Geometry check sheet. Reference: the model listing, model coordinates, mm. A direction names the side the tool comes from. Give positions to 0.01 mm unless a question says otherwise; leave off trailing zeros. Order: outer loops, then holes, each group sorted by start corner. A loop starts at its lowest first (then second) coordinate and runs counter-clockwise, first axis right, second up. Notation, with made-up numbers: M 53,-26 L 87,-26 A12 cw 87,-15 Z; hole C 56.5,71.5 d10. An arc over 180 degrees is marked long. One line per question, with ' | ' between items. Start each with the question number.
from build123d import *
from build123d.topology import SkipClean

# Parameters (mm, degrees)
EXTRUDE_1_DEPTH     = 3
SKETCH_4_W          = 70
SKETCH_4_H          = 3
EXTRUDE_2_DEPTH     = 9
CUT_EXTRUDE_1_REACH = 88.319
FILLET_1_R          = 1
EXTRUDE_3_DEPTH     = 2


with BuildPart() as part:
    # ｽｹｯﾁ2 → ﾎﾞｽ - 押し出し1 (new body)
    with BuildSketch(Plane(origin=(0, 0, 0), x_dir=(1, 0, 0), z_dir=(0, 1, 0))):
        with BuildLine():
            Line((70, 7.6), (40, 7.6))
            Line((40, 7.6), (40, 4.4))
            Line((40, 4.4), (70, 4.4))
            Line((70, 4.4), (84.5, 4.4))
            ThreePointArc((84.5, 4.4), (84.853553391, 4.253553391), (85, 3.9))
            Line((85, 3.9), (85, 0.5))
            ThreePointArc((85, 0.5), (84.853553391, 0.146446609), (84.5, 0))
            Line((84.5, 0), (83.316300355, 0))
            ThreePointArc((83.316300355, 0), (77.25, 2), (71.183699645, 0))
            Line((71.183699645, 0), (70, 0))
            Line((70, 0), (62, 0))
            Line((62, 0), (62, -0.949194177))
            ThreePointArc((62, -0.949194177), (61.80461807, -1.345688605), (61.371168675, -1.432311647))
            Line((61.371168675, -1.432311647), (56, 0))
            Line((56, 0), (0.5, 0))
            ThreePointArc((0.5, 0), (0.146446609, 0.146446609), (0, 0.5))
            Line((0, 0.5), (0, 11.5))
            ThreePointArc((0, 11.5), (0.146446609, 11.853553391), (0.5, 12))
            Line((0.5, 12), (70, 12))
            Line((70, 12), (71.183699645, 12))
            ThreePointArc((71.183699645, 12), (77.25, 10), (83.316300355, 12))
            Line((83.316300355, 12), (84.5, 12))
            ThreePointArc((84.5, 12), (84.853553391, 11.853553391), (85, 11.5))
            Line((85, 11.5), (85, 8.1))
            ThreePointArc((85, 8.1), (84.853553391, 7.746446609), (84.5, 7.6))
            Line((84.5, 7.6), (70, 7.6))
        make_face()
    extrude(amount=EXTRUDE_1_DEPTH)

    # ｽｹｯﾁ4 → ﾎﾞｽ - 押し出し2 (add)
    with BuildSketch(Plane(origin=(0, 3, 0), x_dir=(1, 0, 0), z_dir=(0, 1, 0))):
        with Locations((35, 9.1)):
            Rectangle(SKETCH_4_W, SKETCH_4_H)
    extrude(amount=EXTRUDE_2_DEPTH)

    # ｽｹｯﾁ5 → ｶｯﾄ - 押し出し1 (cut, up to next)
    with BuildSketch(Plane.XY.offset(-7.6), mode=Mode.PRIVATE) as cut_extrude_1_sk1:
        with BuildLine():
            ThreePointArc((64.370652174, 9.924925734), (63.8, 8.7), (64.370652174, 7.475074266))
            ThreePointArc((64.370652174, 7.475074266), (64.782233047, 6.932233047), (65.325074266, 6.520652174))
            ThreePointArc((65.325074266, 6.520652174), (66.55, 5.95), (67.774925734, 6.520652174))
            ThreePointArc((67.774925734, 6.520652174), (68.317766953, 6.932233047), (68.729347826, 7.475074266))
            ThreePointArc((68.729347826, 7.475074266), (69.3, 8.7), (68.729347826, 9.924925734))
            ThreePointArc((68.729347826, 9.924925734), (68.317766953, 10.467766953), (67.774925734, 10.879347826))
            ThreePointArc((67.774925734, 10.879347826), (66.55, 11.45), (65.325074266, 10.879347826))
            ThreePointArc((65.325074266, 10.879347826), (64.782233047, 10.467766953), (64.370652174, 9.924925734))
        make_face()
    cut_extrude_1_tool1 = extrude(cut_extrude_1_sk1.sketch, amount=-CUT_EXTRUDE_1_REACH, mode=Mode.PRIVATE) & part.part
    # ｽｹｯﾁ5 → ｶｯﾄ - 押し出し1 (cut, up to next)
    with BuildSketch(Plane.XY.offset(-7.6), mode=Mode.PRIVATE) as cut_extrude_1_sk2:
        with BuildLine():
            ThreePointArc((5.629347826, 7.475074266), (6.2, 8.7), (5.629347826, 9.924925734))
            ThreePointArc((5.629347826, 9.924925734), (5.217766953, 10.467766953), (4.674925734, 10.879347826))
            ThreePointArc((4.674925734, 10.879347826), (3.45, 11.45), (2.225074266, 10.879347826))
            ThreePointArc((2.225074266, 10.879347826), (1.682233047, 10.467766953), (1.270652174, 9.924925734))
            ThreePointArc((1.270652174, 9.924925734), (0.7, 8.7), (1.270652174, 7.475074266))
            ThreePointArc((1.270652174, 7.475074266), (1.682233047, 6.932233047), (2.225074266, 6.520652174))
            ThreePointArc((2.225074266, 6.520652174), (3.45, 5.95), (4.674925734, 6.520652174))
            ThreePointArc((4.674925734, 6.520652174), (5.217766953, 6.932233047), (5.629347826, 7.475074266))
        make_face()
    cut_extrude_1_tool2 = extrude(cut_extrude_1_sk2.sketch, amount=-CUT_EXTRUDE_1_REACH, mode=Mode.PRIVATE) & part.part
    add(cut_extrude_1_tool1.solids().sort_by_distance((66.55, 8.7, -7.6))[0], mode=Mode.SUBTRACT)
    add(cut_extrude_1_tool2.solids().sort_by_distance((3.45, 8.7, -7.6))[0], mode=Mode.SUBTRACT)

    # ﾌｨﾚｯﾄ1
    fillet_1_edges = [part.edges().sort_by_distance(p)[0] for p in [
        (70, 12, -9.1),
        (0, 12, -9.1),
    ]]
    fillet(fillet_1_edges, radius=FILLET_1_R)

    # ｽｹｯﾁ6 → ﾎﾞｽ - 押し出し3 (add)
    with SkipClean():  # the faces are left unmerged after this step: merging them gives an invalid solid
        with BuildSketch(Plane.XY.offset(-7.6)):
            with BuildLine():
                Line((1.85, 9.85), (1.85, 7.55))
                ThreePointArc((1.85, 7.55), (1.946690123, 7.002223209), (2.225074266, 6.520652174))
                ThreePointArc((2.225074266, 6.520652174), (1.682233047, 6.932233047), (1.270652174, 7.475074266))
                ThreePointArc((1.270652174, 7.475074266), (0.7, 8.7), (1.270652174, 9.924925734))
                ThreePointArc((1.270652174, 9.924925734), (1.682233047, 10.467766953), (2.225074266, 10.879347826))
                ThreePointArc((2.225074266, 10.879347826), (1.946690123, 10.397776791), (1.85, 9.85))
            make_face()
            with BuildLine():
                Line((5.05, 9.85), (5.05, 7.55))
                ThreePointArc((5.05, 7.55), (4.953309877, 7.002223209), (4.674925734, 6.520652174))
                ThreePointArc((4.674925734, 6.520652174), (5.217766953, 6.932233047), (5.629347826, 7.475074266))
                ThreePointArc((5.629347826, 7.475074266), (6.2, 8.7), (5.629347826, 9.924925734))
                ThreePointArc((5.629347826, 9.924925734), (5.217766953, 10.467766953), (4.674925734, 10.879347826))
                ThreePointArc((4.674925734, 10.879347826), (4.953309877, 10.397776791), (5.05, 9.85))
            make_face()
            with BuildLine():
                Line((64.95, 9.85), (64.95, 7.55))
                ThreePointArc((64.95, 7.55), (65.046690123, 7.002223209), (65.325074266, 6.520652174))
                ThreePointArc((65.325074266, 6.520652174), (64.782233047, 6.932233047), (64.370652174, 7.475074266))
                ThreePointArc((64.370652174, 7.475074266), (63.8, 8.7), (64.370652174, 9.924925734))
                ThreePointArc((64.370652174, 9.924925734), (64.782233047, 10.467766953), (65.325074266, 10.879347826))
                ThreePointArc((65.325074266, 10.879347826), (65.046690123, 10.397776791), (64.95, 9.85))
            make_face()
            with BuildLine():
                Line((68.15, 9.85), (68.15, 7.55))
                ThreePointArc((68.15, 7.55), (68.053309877, 7.002223209), (67.774925734, 6.520652174))
                ThreePointArc((67.774925734, 6.520652174), (68.317766953, 6.932233047), (68.729347826, 7.475074266))
                ThreePointArc((68.729347826, 7.475074266), (69.3, 8.7), (68.729347826, 9.924925734))
                ThreePointArc((68.729347826, 9.924925734), (68.317766953, 10.467766953), (67.774925734, 10.879347826))
                ThreePointArc((67.774925734, 10.879347826), (68.053309877, 10.397776791), (68.15, 9.85))
            make_face()
        extrude(amount=-EXTRUDE_3_DEPTH)


solid = part.part
Item 1: Material ranges on line 1 along X through (y, z) = (9.25, -8.5); line 2 along X through (y, z) = (10, -9.5); line 3 along Z through (x, y) = (48, 1.75), recorded low to high.
Item 2: Cross-section at B-B, the plane y = 8.5. Record the cut outline in (x, z), plus the area to 3 significant figures.
Item 3: Cross-section at A-A, the plane x = 50. Record the cut outline in (y, z), plus the area to 3 significant figures.
Item 4: Cross-section at D-D, the plane z = -3. Record the cut outline in (x, y).
Item 5: Depth check by flat-ended pin: pin 1 (3.5 mm diameter, centred on y = 7.5, z = -9.5, fed in from +X); pin 2 (1.7 mm diameter, centred on x = 1.5, y = 8, fed in from -Z); pin 3 (0.8 mm diameter, centred on y = 1, z = 0.5, fed in from +X); pin 4 (5 mm diameter, centred on y = 7.5, z = -1, fed in from +X). Enter the tip coordinate at first touch or a pass-through.
Item 6: Cross-section at C-C, the plane x = 39. Record the cut outline in (y, z), plus the area to 3 significant figures.
Item 7: Set-up check for faces 5 (the flat face through (5.05, 9, -9)), 6 (the flat face through (43, 6, -7.6)), 7 (the flat face through (35, 7, -10.6)): record each of +Z, -Z, +X, -X, +Y, -Y from which the full face is reachable in a straight line by a thin tool's end or side.
Item 8: Mould release check, pull along Y, two halves, no side actions. Record for faces 1 (the flat face through (43, 0, -4)), 2 (the flat face through (40, 1, -6)), 3 (the flat face through (64.6, 8.7, -9.6)), 4 (the flat face through (53, 3, -11)): released by +Y, released by -Y, zero draft, split by the parting line, or undercut.
Outcome:
1) line 1: x = 0 to 1.85, 5.05 to 64.95, 68.15 to 70 | line 2: x = 0 to 1.86, 5.04 to 64.96, 68.14 to 70 | line 3: z = -12 to -7.6, -4.4 to 0
2) outline: M 0,-10.6 L 0.71,-10.6 L 0.71,-9.6 L 1.85,-9.6 L 1.85,-7.6 L 0,-7.6 Z; M 5.05,-9.6 L 6.19,-9.6 L 6.19,-10.6 L 63.81,-10.6 L 63.81,-9.6 L 64.95,-9.6 L 64.95,-7.6 L 5.05,-7.6 Z; M 68.15,-9.6 L 69.29,-9.6 L 69.29,-10.6 L 70,-10.6 L 70,-7.6 L 68.15,-7.6 Z | area: 186 mm²
3) outline: M 0,-12 L 3,-12 L 3,-10.6 L 12,-10.6 L 12,-7.6 L 0,-7.6 Z; M 0,-4.4 L 3,-4.4 L 3,0 L 0,0 Z | area: 53.4 mm²
4) outline: M 0,0 L 85,0 L 85,3 L 0,3 Z
5) pin 1: stops at x = 70 | pin 2: stops at z = -10.6 | pin 3: stops at x = 62 | pin 4: passes through
6) outline: M 0,-12 L 3,-12 L 3,-10.6 L 12,-10.6 L 12,-7.6 L 3,-7.6 L 3,0 L 0,0 Z | area: 63.0 mm²
7) face 5: +Z, -Z | face 6: +X, +Y | face 7: -Z, +X, -X, +Y
8) face 1: released by -Y | face 2: zero draft | face 3: undercut | face 4: released by +Y
